Input: dimensioned drawing with shaded views. Units: mm. Origin: part minimum x, y, z. A direction names the side the tool comes from. Give positions to 0.01 mm unless a question says otherwise; leave off trailing zeros. Loops run counter-clockwise (first coordinate to the right, second up) from the corner with the lowest first, then second, coordinate; pieces in that order, holes last.
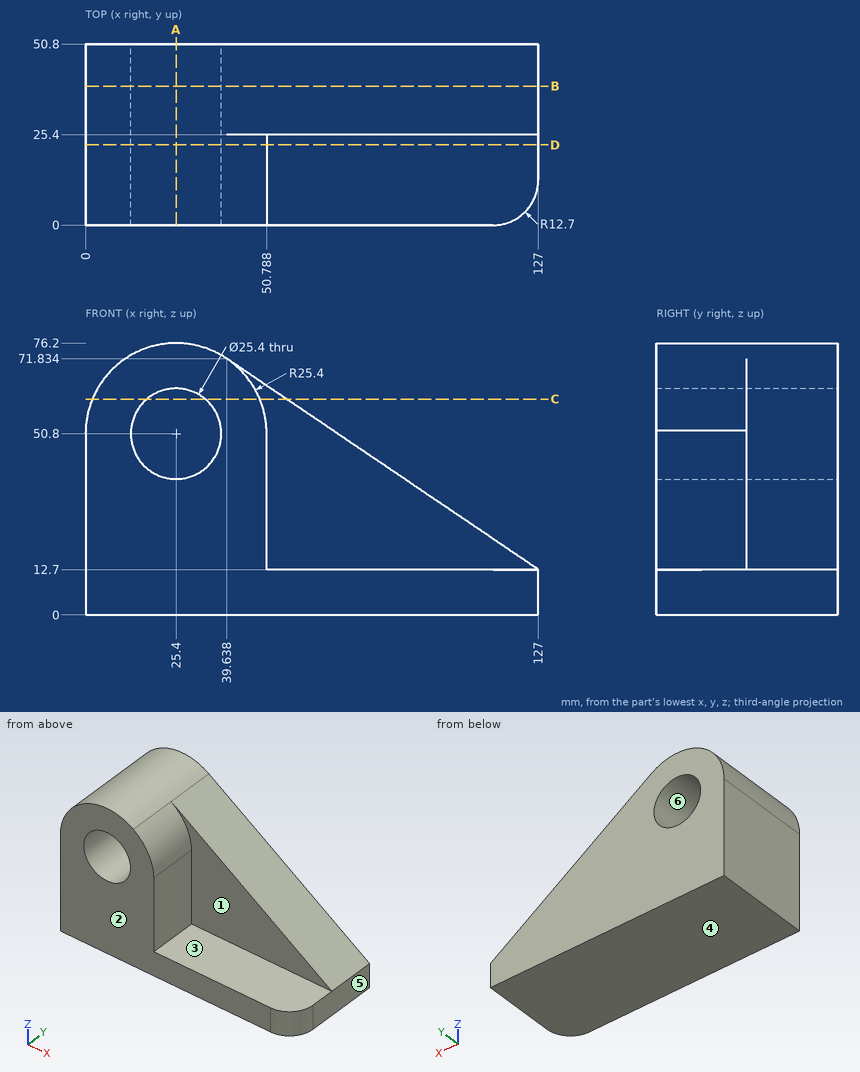
(1) Reachability of the marked faces 1 and 2 from +Z, -Z, +X, -X, +Y, -Y: full face, straight path, thin tool, end or side. Return the list, or none.
A:
face 1: +Z, +X, -Y
face 2: +Z, -Z, +X, -X, -Y
(2) Section A-A, the plane x = 25.4. Return the cut outline in (y, z), then the cut area to 3 significant figures.
A:
outline: (0, 0) - (50.8, 0) - (50.8, 38.1) - (0, 38.1) - close; (0, 63.5) - (50.8, 63.5) - (50.8, 76.2) - (0, 76.2) - close
area: 2,580 mm2
(3) Section B-B, the plane y = 39. Return the cut outline in (x, z).
A:
outline: (0, 0) - (127, 0) - (127, 12.7) - (39.64, 71.83) arc R25.4 ccw to (0, 50.8) - close; hole circle Ø25.4 at (25.4, 50.8)
(4) First-contact query: pin 1 (17.5 mm diameter, centred on x = 70, z = 39.5, fed in from -Y); pin 2 (12.5 mm diameter, centred on x = 104, y = 15.5, fed in from +Z); pin 3 (10 mm diameter, centred on x = 19, y = 44, fed in from +Z). Flat tips, straight axial feed; report the tip coordinate or a pass-through.
A:
pin 1: stops at y = 25.4
pin 2: stops at z = 12.7
pin 3: stops at z = 76.16
(5) Section D-D, the plane y = 22.5. Return the cut outline in (x, z), then the cut area to 3 significant figures.
A:
outline: (0, 0) - (127, 0) - (127, 12.7) - (50.79, 12.7) - (50.79, 51.59) arc R25.4 ccw to (0, 50.8) - close; hole circle Ø25.4 at (25.4, 50.8)
area: 4,050 mm2
(6) Mould query, pull axis Z, two halves, no side actions, for the marked faces 3, 4, 5 and 6. Classes: pulls with the +Z half, pulls with the -Z half, needs draft (parallel to the pull), parting line crosses it, or undercut.
A:
face 3: pulls with the +Z half
face 4: pulls with the -Z half
face 5: needs draft
face 6: undercut
(7) Ray query, line 1 along Z through (x, y) = (25.4, 20.5); line 2 along X through (y, z) = (19, 50) (1 decimal); line 3 along Z through (x, y) = (86.5, 17). Return the intervals inside material, ascending.
A:
line 1: z = 0 to 38.1, 63.5 to 76.2
line 2: x = 0 to 12.7, 38.1 to 50.8
line 3: z = 0 to 12.7
(8) Section C-C, the plane z = 60.5. Return the cut outline in (x, y) (1 decimal), then the cut area to 3 significant figures.
A:
outline: (1.9, 0) - (17.2, 0) - (17.2, 50.8) - (1.9, 50.8) - close; (33.6, 0) - (48.9, 0) - (48.9, 25.4) - (56.4, 25.4) - (56.4, 50.8) - (33.6, 50.8) - close
area: 1,740 mm2
